Work out the finished part from the listing and answer in its coordinate system (mm). Face numbers are marked on the shaded views. Give positions to 0.01 mm unless a question says otherwise; leave off trailing zeros. Use CSV: the item, a comma, the result in double quotes.
from build123d import *

# Parameters (mm, degrees)
FILLET1_R                  = 0.5
FILLET5_R                  = 5
SKETCH12_R                 = 86
SKETCH12_R_2               = 55
BOSS_EXTRUDE1_DEPTH        = 13.35
M14X2_0_TAPPED_HOLE2_D     = 12
M14X2_0_TAPPED_HOLE2_DEPTH = 16
M14X2_0_TAPPED_HOLE2_TIP   = 3.605163714


with BuildPart() as part:
    # Sketch1 → Revolve1 (revolve)
    with BuildSketch(Plane(origin=(0, 0, 0), x_dir=(1, 0, 0), z_dir=(0, 1, 0)), mode=Mode.PRIVATE) as revolve1_sk:
        with BuildLine():
            Line((0.595225647, 30), (2.595225647, 30))
            Line((2.595225647, 30), (2.595225647, 48))
            ThreePointArc((2.595225647, 48), (3.181012085, 49.414213562), (4.595225647, 50))
            Line((4.595225647, 50), (6.595225647, 50))
            Line((6.595225647, 50), (6.595225647, 55))
            Line((6.595225647, 55), (1.744360585, 55))
            Line((1.744360585, 55), (1.744360585, 86))
            Line((1.744360585, 86), (-2.255639415, 86))
            Line((-2.255639415, 86), (-2.255639415, 49))
            ThreePointArc((-2.255639415, 49), (-3.134319072, 46.878679656), (-5.255639415, 46))
            Line((-5.255639415, 46), (-6.404774353, 46))
            Line((-6.404774353, 46), (-6.404774353, 36))
            Line((-6.404774353, 36), (0.595225647, 36))
            Line((0.595225647, 36), (0.595225647, 30))
        make_face()
    revolve(revolve1_sk.sketch.rotate(Axis((0, 0, 0), (1, 0, 0)), 180), axis=Axis((0, 0, 0), (1, 0, 0)))

    # Fillet1
    fillet1_edges = [part.edges().sort_by_distance(p)[0] for p in [
        (-6.404774353, 0, -36),
    ]]
    fillet(fillet1_edges, radius=FILLET1_R)

    # Fillet5
    # the kernel refuses this fillet: 5 mm, written as the material it takes off along each edge
    with BuildSketch(Plane(origin=(-2.255639415, 0, 0), x_dir=(0, 0, 1), z_dir=(0, 1, 0))) as fillet5_piece_1:
        with BuildLine():
            CenterArc((81.101020514, 5), FILLET5_R, 270, 78.463040967)
            Line((86, 4), (86.09797959, 3.98))
            ThreePointArc((86.09797959, 3.98), (86.1, 2), (86.1, 0))
            Line((86.1, 0), (86, -0.1))
            Line((86, -0.1), (81.101020514, -0.1))
            Line((81.101020514, -0.1), (81.101020514, 0))
        make_face()
    revolve(axis=Axis((-2.255639415, 0, 0), (1, 0, 0)), mode=Mode.SUBTRACT)

    # Sketch12 → Boss-Extrude1 (add)
    with BuildSketch(Plane(origin=(1.744360585, 0, 0), x_dir=(0, 0, -1), z_dir=(1, 0, 0))):
        Circle(SKETCH12_R)
        with Locations(Location((0, 0, 0), (0, 0, 180))):
            Circle(SKETCH12_R_2, mode=Mode.SUBTRACT)
    extrude(amount=BOSS_EXTRUDE1_DEPTH)

    # M14x2.0 Tapped Hole2
    with Locations(Plane.ZY.offset(2.255639415)):
        with Locations((-56.335394412, 32.575765386), (0, 65.050510257), (56.291651246, 32.5), (56.24790808, -32.525255129), (-0.087486332, -65), (-56.379137578, -32.449489743)):
            Hole(M14X2_0_TAPPED_HOLE2_D / 2, depth=M14X2_0_TAPPED_HOLE2_DEPTH)
            with Locations((0, 0, -(M14X2_0_TAPPED_HOLE2_DEPTH + M14X2_0_TAPPED_HOLE2_TIP / 2))):  # 118° drill point
                Cone(0, M14X2_0_TAPPED_HOLE2_D / 2, M14X2_0_TAPPED_HOLE2_TIP, mode=Mode.SUBTRACT)


solid = part.part
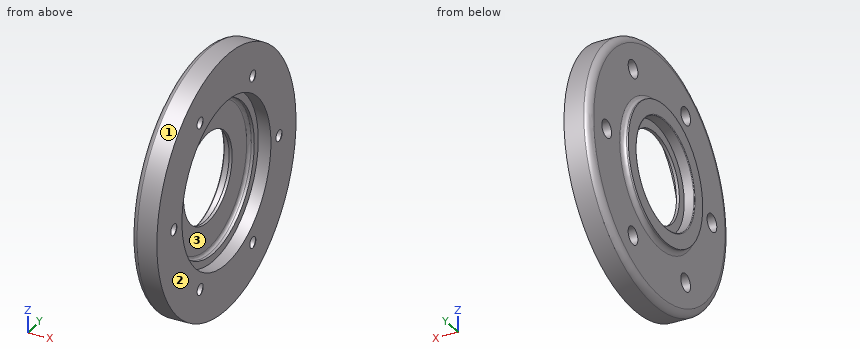
Item 1: Find the intervals of material crossed by line 1 (Y direction, x = 2.1, z = 0); line 2 (Y direction, x = 5.4, z = 0); line 3 (Y direction, x = 6.75, z = -60), in increasing order.
Determined:
line 1,"y = -86 to -71, -59 to -30, 30 to 59.05, 71.05 to 86"
line 2,"y = -86 to -71, -59 to -50, 50 to 59.05, 71.05 to 86"
line 3,"y = -61.61 to -37.23, -27.67 to 27.82, 37.33 to 61.61"
Item 2: Given P1, Ø11, axis at y = -32.53, z = 56.25, coming from the -X side; P2, Ø1, axis at x = 10, z = 14, coming from the -Y side; P3, Ø2, axis at x = 6, y = -28, coming from the +Z side, each flat-ended and moving along its own axis, determine where each tip first touches the part or whether it passes through.
Determined:
P1,"stops at x = 14.04"
P2,"stops at y = -84.93"
P3,"stops at z = 81.65"
Item 3: The mould has two halves that part along Z. Classify the marked faces 1, 2 and 3: pulls with the +Z half, pulls with the -Z half, needs draft (parallel to the pull), parting line crosses it, or undercut.
Determined:
face 1,"parting line crosses it"
face 2,"needs draft"
face 3,"undercut"
Item 4: A cutting plane is placed at B-B on z = 0. State how many separate pieces and enclosed holes the cut face has, and give its area (3 significant figures).
Determined:
separate pieces,"4"
enclosed holes,"0"
area,"992 mm²"
